For this review, take the finished solid that the model builds, in its own axes (mm). A direction names the side the tool comes from. Round coordinates to 2 decimals unless told otherwise and drop trailing zeros. Order: outer loops, then holes, each group sorted by start corner. A loop starts at its lowest first (then second) coordinate and runs counter-clockwise, first axis right, second up. Notation, with made-up numbers: M 5,17 L 45,17 A11 cw 45,23 Z; hole C 30,79 d5. An arc over 180 degrees is marked long. Answer as a JSON object with one key per item and string values.
from build123d import *

# Parameters (mm, degrees)
SKETCH3_R           = 9
SKETCH3_R_2         = 7
BOSS_EXTRUDE1_DEPTH = 0.8


with BuildPart() as part:
    # Sketch2 → Revolve1 (revolve)
    with BuildSketch(Plane(origin=(0, 0, 0), x_dir=(0, 0, -1), z_dir=(1, 0, 0)), mode=Mode.PRIVATE) as revolve1_sk:
        Polygon((-16, 11), (-10.2, 11), (-10.2, 9), (16, 9), (16, 7), (-12.2, 7), (-12.2, 9), (-16, 9), align=None)
    revolve(revolve1_sk.sketch.rotate(Axis((0, 0, 152.237580052), (0, 0, -1)), 90), axis=Axis((0, 0, 152.237580052), (0, 0, -1)))  # turned: the seam where the file's is

    # Sketch3 → Boss-Extrude1 (add)
    with BuildSketch(Plane.XY.offset(12.2)):
        Circle(SKETCH3_R)
        Circle(SKETCH3_R_2, mode=Mode.SUBTRACT)
    extrude(amount=BOSS_EXTRUDE1_DEPTH)


solid = part.part
1) Mouldability with a two-part tool opening along X and no side actions: class faces 4 (the cylindrical face through (-2.38, 10.74, 13.06)), 5 (the flat face through (2, 9, 10.2)), 6 (the cylindrical face through (-6.633, -6.083, 14.521)), 7 (the cylindrical face through (6.466, -2.681, -1.703)) as +X half, -X half, draft (parallel to the pull), parting line (faces both ways), or undercut.
Geometry check:
{"face 4": "parting line", "face 5": "draft", "face 6": "undercut", "face 7": "undercut"}
2) Machinability: for faces 1 (the flat face through (0, 7.3, -16)), 2 (the flat face through (0, -7.3, 13)), 3 (the cylindrical face through (-6.633, -6.083, -3.083)), which of the approach directions +Z, -Z, +X, -X, +Y, -Y give a long, thin tool a straight path to every point of the face, cutting with its end or side? Answer none if there is none.
Geometry check:
{"face 1": "-Z, +X, -X, +Y, -Y", "face 2": "+Z", "face 3": "-Z"}
3) Add section C-C on z = -10. State the section outline as (x, y) points.
Geometry check:
{"outline": "C 0,0 d18; hole C 0,0 d14"}
4) Insertion check: P1, Ø1, axis at x = 7, y = -2.5, coming from the +Z side; P2, Ø5.5, axis at x = -3.5, y = 0.5, coming from the +Z side; P3, Ø1, axis at y = 5, z = -11.5, coming from the -X side; P4, Ø5, axis at x = 0, z = -7, coming from the -Y side. Each pin has a flat end and moves straight along its axis. Give the tip position at first contact, or say it passes through.
Geometry check:
{"P1": "stops at z = 13", "P2": "passes through", "P3": "stops at x = -7.79", "P4": "stops at y = -9"}
5) For L1, parallel to Y at x = 0, z = 13.8; L2, parallel to Y at x = 0, z = -7.75; L3, parallel to Z at x = 9.25, y = 1, list the stretches that pass through material, from the lowest coordinate up.
Geometry check:
{"L1": "y = -11 to -9, 9 to 11", "L2": "y = -9 to -7, 7 to 9", "L3": "z = 10.2 to 16"}
6) Add section A-A on x = 0. State the section outline as (y, z) points, and give its area (3 significant figures).
Geometry check:
{"outline": "M -11,10.2 L -9,10.2 L -9,-16 L -7,-16 L -7,13 L -9,13 L -9,16 L -11,16 Z; M 7,-16 L 9,-16 L 9,10.2 L 11,10.2 L 11,16 L 9,16 L 9,13 L 7,13 Z", "area": "139 mm²"}
7) Add section D-D on y = 9.5. State the section outline as (x, z) points.
Geometry check:
{"outline": "M -5.55,10.2 L 5.55,10.2 L 5.55,16 L -5.55,16 Z"}
